from build123d import *

# Parameters (mm, degrees)
F0_W     = 101.6
F0_H     = 101.6
F1_DEPTH = 101.6
F2_R     = 6.552167
F3_DEPTH = 101.6
F4_W     = 50.8
F4_H     = 50.8
F5_DEPTH = 50.8


with BuildPart() as f1:
    # F0 (on Front) → F1 (new body)
    with BuildSketch(Plane.XZ):
        with Locations((-50.8, 50.8)):
            Rectangle(F0_W, F0_H)
    extrude(amount=F1_DEPTH)

    # F2 (on face) → F3 (cut)
    with BuildSketch(Plane.XY.offset(101.6)):
        with Locations((-94.014853, -7.79883)):
            Circle(F2_R)
    extrude(amount=-F3_DEPTH, mode=Mode.SUBTRACT)

    # F4 (on face) → F5 (cut)
    with BuildSketch(Plane.XY.offset(101.6)):
        with Locations((-25.4, -76.2)):
            Rectangle(F4_W, F4_H)
    extrude(amount=-F5_DEPTH, mode=Mode.SUBTRACT)


solid = f1.part
Work out the finished part from the listing and answer in its coordinate system (mm). A direction names the side the tool comes from. Coordinates: 2 decimals unless noted, no trailing zeros. Write each loop counter-clockwise with the first axis right and the second up, starting at its lowest first coordinate (ties: lowest second). Pieces come first, ordered by that corner, then holes. Notation, with made-up numbers: M 72.5,-34.5 L 103.5,-34.5 A25 ccw 103.5,-9.5 Z; hole C 85.25,7.25 d6. An arc over 180 degrees is marked long. Use one line per item in the form item = value. Start each with the question number.
1. The part is cut by section C-C (z = 73). Give the vertices of the cut face in (x, y).
2. The part is cut by section A-A (x = -93). Give the vertices of the cut face in (y, z), plus the area to 3 significant figures.
3. This flat-tipped pin is pushed along its axis until it touches: P1, Ø17, axis at x = -94.01, y = -7.8, coming from the -Z side. Where does it stop, or does it pass through?
4. A tool of negligible diameter and unlimited length cuts with its end or side. For faces 5 (the face through (-63, -39, 101.6)), 6 (the face through (-26, -76, 50.8)), from which of +Z, -Z, +X, -X, +Y, -Y can it reach the whole face along a straight path? Write none if from no direction.
5. Straight lines are drawn through the part: probe 1 along Z at (x, y) = (-11.5, -67); probe 2 along X at (y, z) = (-78, 65); probe 3 along Y at (x, z) = (-40, 87.5). For each, find the intervals that lie inside material, in ascending order. Write a range as from..to.
6. The mould has two halves that part along X. Classify faces 1 (the face through (-63, -101.6, 40)), 2 (the face through (-50.8, -77, 77)), 3 (the face through (-87.765, -5.831, 51.511)), 4 (the face through (-101.6, -50, 50)): released by +X, released by -X, zero draft, split by the parting line, or undercut.
7. The part is cut by section B-B (y = -66.5). Give the vertices of the cut face in (x, z).
8. The part is cut by section D-D (x = -20.5). Give the vertices of the cut face in (y, z), plus the area to 3 significant figures.
Evaluation:
q1.outline = M -101.6,-101.6 L -50.8,-101.6 L -50.8,-50.8 L 0,-50.8 L 0,0 L -101.6,0 Z; hole C -94.01,-7.8 d13.1
q2.outline = M -101.6,0 L -14.27,0 L -14.27,101.6 L -101.6,101.6 Z; M -1.33,0 L 0,0 L 0,101.6 L -1.33,101.6 Z
q2.area = 9,010 mm^2
q3.P1 = 0
q4.face_5 = +Z, +X, -X, +Y, -Y
q4.face_6 = +Z, +X, -Y
q5.probe_1 = 0..50.8
q5.probe_2 = -101.6..-50.8
q5.probe_3 = -50.8..0
q6.face_1 = zero draft
q6.face_2 = released by +X
q6.face_3 = undercut
q6.face_4 = released by -X
q7.outline = M -101.6,0 L 0,0 L 0,50.8 L -50.8,50.8 L -50.8,101.6 L -101.6,101.6 Z
q8.outline = M -101.6,0 L 0,0 L 0,101.6 L -50.8,101.6 L -50.8,50.8 L -101.6,50.8 Z
q8.area = 7,740 mm^2
